The listing builds one solid part. Answer for the finished solid, in the listing's coordinates (mm). Face numbers are marked on the shaded views. A direction names the side the tool comes from. Give positions to 0.01 mm unless a question says otherwise; leave off trailing zeros. Loops run counter-clockwise (first coordinate to the right, second up) from the corner with the lowest first, then second, coordinate; pieces in that order, holes last. Notation, with made-up numbers: M -0.75,-22 L 53.25,-22 A34 cw 53.25,14 Z; hole C 1,-24.75 d7. An arc over 180 degrees is marked long. One line per item, written item: value. Start each with the question number.
Q1. The mould has two halves that part along X. Classify the marked faces 3, 4 and 5: +X half, -X half, draft (parallel to the pull), parting line (faces both ways), or undercut.
Q2. For the marked faces 1 and 2, determine the directions among +Z, -Z, +X, -X, +Y, -Y from which every point of the face is accessible in a straight line to the end or side of a thin tool.
Q3. Consider L1, parallel to Z at x = 6.5, y = 2.5; L2, parallel to X at y = 2.3, z = 1; L3, parallel to X at y = 0.5, z = 9. Determine where each line is inside the solid, lowest interval first.
Q4. Flat-ended cylindrical pins translate along their axes: pin 1 (1.5 mm diameter, centred on x = 4, y = 2, fed in from +Z); pin 2 (1 mm diameter, centred on x = 6.5, y = 0.5, fed in from +Z); pin 3 (2 mm diameter, centred on x = 0, z = 0, fed in from +Y); pin 4 (8 mm diameter, centred on x = -5.5, z = -6.5, fed in from -Y). Find the tip coordinate at first contact, or state that the pin passes through.
Q5. A cutting plane is placed at A-A, the plane y = 0.8. State how many separate pieces and enclosed holes the cut face has, and give its area (3 significant figures).
Q6. A cutting plane is placed at C-C, the plane x = -12.5. Determine the outline of the cut face in (y, z).
Q7. A cutting plane is placed at B-B, the plane z = -9.5. Determine the outline of the cut face in (x, y), and give its area (3 significant figures).
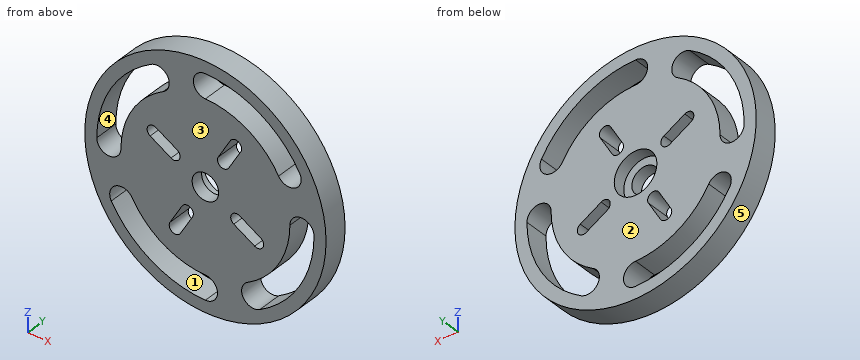
from build123d import *

# Parameters (mm, degrees)
SKETCH_1_R          = 15
SKETCH_1_R_2        = 2.65
SKETCH_1_R_3        = 1.65
EXTRUDE_2_DEPTH     = 3
SKETCH_2_R          = 1.65
CUT_EXTRUDE_2_DEPTH = 17
SKETCH_2_4_R        = 2.65
SKETCH_2_4_R_2      = 1.65
CUT_EXTRUDE_3_DEPTH = 1.5


with BuildPart() as part:
    # Sketch 1 → Extrude 2 (new body)
    with BuildSketch(Plane(origin=(0, 0, 0), x_dir=(1, 0, 0), z_dir=(0, 1, 0))):
        Circle(SKETCH_1_R)
        Circle(SKETCH_1_R_2, mode=Mode.SUBTRACT)
        Circle(SKETCH_1_R_2)
        Circle(SKETCH_1_R_3, mode=Mode.SUBTRACT)
        Circle(SKETCH_1_R_3)
    extrude(amount=EXTRUDE_2_DEPTH)

    # Sketch 2 → Cut-Extrude 2 (cut)
    with BuildSketch(Plane(origin=(0, 3, 0), x_dir=(1, 0, 0), z_dir=(0, 1, 0))):
        with BuildLine():
            ThreePointArc((13.504705492, 0), (11.694050248, 6.754721254), (6.747614899, 11.698152145))
            ThreePointArc((6.747614899, 11.698152145), (4.698799352, 11.14828411), (5.248667387, 9.099468564))
            ThreePointArc((5.248667387, 9.099468564), (9.096277882, 5.254195103), (10.504705492, 0))
            ThreePointArc((10.504705492, 0), (12.004705492, -1.5), (13.504705492, 0))
        make_face()
        with BuildLine():
            ThreePointArc((0, -13.504705492), (6.754721254, -11.694050248), (11.698152145, -6.747614899))
            ThreePointArc((11.698152145, -6.747614899), (11.14828411, -4.698799352), (9.099468564, -5.248667387))
            ThreePointArc((9.099468564, -5.248667387), (5.254195103, -9.096277882), (0, -10.504705492))
            ThreePointArc((0, -10.504705492), (-1.5, -12.004705492), (0, -13.504705492))
        make_face()
        with BuildLine():
            ThreePointArc((0, 13.504705492), (-6.754721254, 11.694050248), (-11.698152145, 6.747614899))
            ThreePointArc((-11.698152145, 6.747614899), (-11.14828411, 4.698799352), (-9.099468564, 5.248667387))
            ThreePointArc((-9.099468564, 5.248667387), (-5.254195103, 9.096277882), (0, 10.504705492))
            ThreePointArc((0, 10.504705492), (1.5, 12.004705492), (0, 13.504705492))
        make_face()
        Circle(SKETCH_2_R)
        with BuildLine():
            ThreePointArc((-13.504705492, 0), (-11.694050248, -6.754721254), (-6.747614899, -11.698152145))
            ThreePointArc((-6.747614899, -11.698152145), (-4.698799352, -11.14828411), (-5.248667387, -9.099468564))
            ThreePointArc((-5.248667387, -9.099468564), (-9.096277882, -5.254195103), (-10.504705492, 0))
            ThreePointArc((-10.504705492, 0), (-12.004705492, 1.5), (-13.504705492, 0))
        make_face()
        with BuildLine():
            Line((-1.601346136, 4.271790088), (-3.101872288, 6.869562454))
            ThreePointArc((-3.101872288, 6.869562454), (-4.126446917, 7.143874008), (-4.400758471, 6.119299378))
            Line((-4.400758471, 6.119299378), (-2.900232319, 3.521527012))
            ThreePointArc((-2.900232319, 3.521527012), (-1.87565769, 3.247215458), (-1.601346136, 4.271790088))
        make_face()
        with BuildLine():
            Line((-4.271790088, -1.601346136), (-6.869562454, -3.101872288))
            ThreePointArc((-6.869562454, -3.101872288), (-7.143874008, -4.126446917), (-6.119299378, -4.400758471))
            Line((-6.119299378, -4.400758471), (-3.521527012, -2.900232319))
            ThreePointArc((-3.521527012, -2.900232319), (-3.247215458, -1.87565769), (-4.271790088, -1.601346136))
        make_face()
        with BuildLine():
            Line((1.601346136, -4.271790088), (3.101872288, -6.869562454))
            ThreePointArc((3.101872288, -6.869562454), (4.126446917, -7.143874008), (4.400758471, -6.119299378))
            Line((4.400758471, -6.119299378), (2.900232319, -3.521527012))
            ThreePointArc((2.900232319, -3.521527012), (1.87565769, -3.247215458), (1.601346136, -4.271790088))
        make_face()
        with BuildLine():
            Line((4.271790088, 1.601346136), (6.869562454, 3.101872288))
            ThreePointArc((6.869562454, 3.101872288), (7.143874008, 4.126446917), (6.119299378, 4.400758471))
            Line((6.119299378, 4.400758471), (3.521527012, 2.900232319))
            ThreePointArc((3.521527012, 2.900232319), (3.247215458, 1.87565769), (4.271790088, 1.601346136))
        make_face()
    extrude(amount=-CUT_EXTRUDE_2_DEPTH, mode=Mode.SUBTRACT)

    # Sketch 2_4 → Cut-Extrude 3 (cut)
    with BuildSketch(Plane(origin=(0, 3, 0), x_dir=(1, 0, 0), z_dir=(0, 1, 0))):
        Circle(SKETCH_2_4_R)
        Circle(SKETCH_2_4_R_2, mode=Mode.SUBTRACT)
    extrude(amount=-CUT_EXTRUDE_3_DEPTH, mode=Mode.SUBTRACT)


solid = part.part
Answer block:
1. face 3: draft
1. face 4: undercut
1. face 5: parting line
2. face 1: +Y, -Y
2. face 2: +Z, -Z, +X, -X, +Y
3. L1: -13.52 to -11.81, -8.25 to -4.5, -2.89 to 8.25, 11.84 to 13.52
3. L2: -14.97 to -13.47, -10.46 to -2.45, 2.45 to 10.89, 13.12 to 14.97
3. L3: -12 to -10.07, -5.42 to 5.42, 10.07 to 12
4. pin 1: z = 14.64
4. pin 2: z = 13.75
4. pin 3: through
4. pin 4: y = 0
5. separate pieces: 1
5. enclosed holes: 9
5. area: 494 mm^2
6. outline: M 0,-8.29 L 3,-8.29 L 3,-1.42 L 0,-1.42 Z; M 0,5.11 L 3,5.11 L 3,8.29 L 0,8.29 Z
7. outline: M -11.61,0 L -9.6,0 L -9.6,3 L -11.61,3 Z; M -4.48,0 L 4.8,0 L 4.8,3 L -4.48,3 Z; M 9.6,0 L 11.61,0 L 11.61,3 L 9.6,3 Z
7. area: 39.9 mm^2
